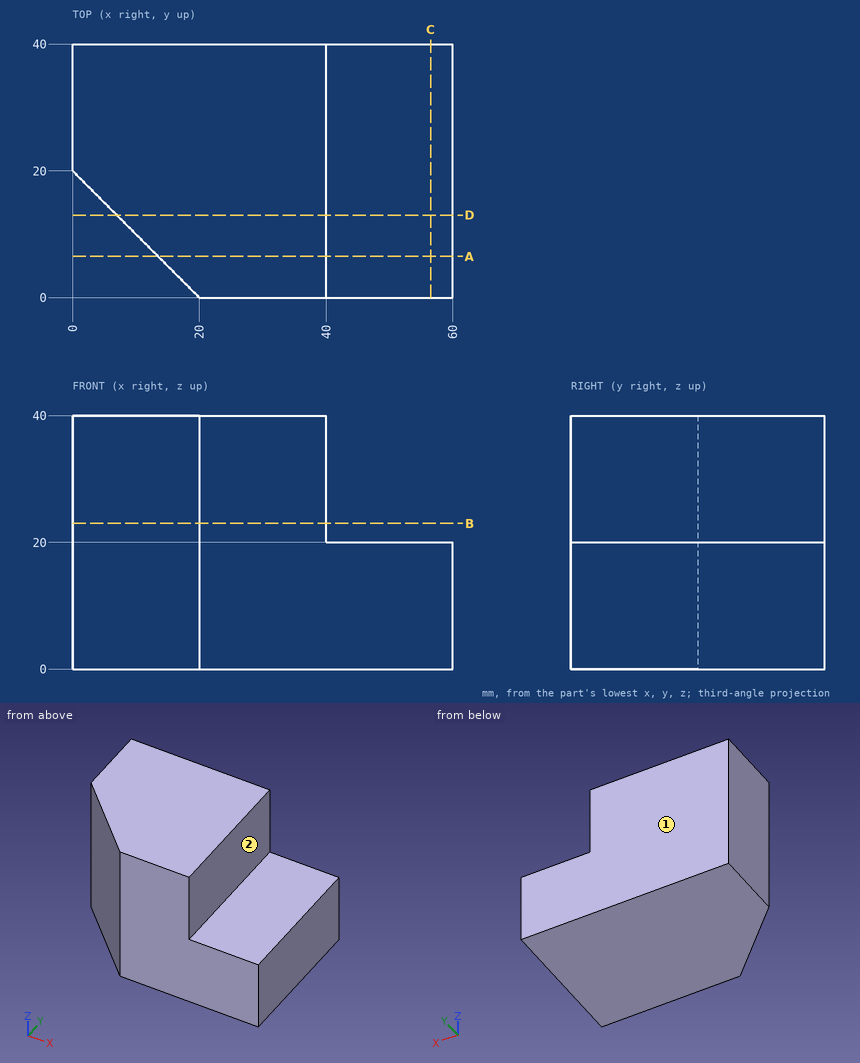
Could you check a few things on this drawing? It's one solid part, dimensions in mm from its lowest x, y, z. A direction names the side the tool comes from. Round coordinates to 2 decimals unless told otherwise and drop trailing zeros. Write each loop counter-clockwise with the first axis right and the second up, starting at its lowest first coordinate (ties: lowest second). Pieces come first, ordered by that corner, then holes. Notation, with made-up numbers: (-11.5, -3.5) -> (12.5, -3.5) arc R34 cw to (12.5, 27.5) -> close; hole circle Ø3 at (4.25, 21.5). An arc over 180 degrees is marked (long way). One line per question, with ' | ' between items. Start each with the question number.
1) I need wall thicknesses on line 1 (Z direction, x = 44, y = 15); line 2 (X direction, y = 33, z = 32); line 3 (Y direction, x = 4.5, z = 4). Which ranges of each line are inside material? Lowest first, please. Write a range as [from, to].
2) Suppose I cut it at A-A on y = 6.5. Write out the boundary of the cut face in (x, z).
3) Suppose I cut it at B-B on z = 23. Write out the boundary of the cut face in (x, y).
4) Suppose I cut it at C-C on x = 56.5. Write out the boundary of the cut face in (y, z), then the cut area to 3 significant figures.
5) I'm going to push flat-ended pins straight in: P1, Ø3, axis at x = 15.5, z = 22.5, coming from the -Y side; P2, Ø6, axis at x = 47, y = 15, coming from the +Z side; P3, Ø2, axis at x = 42.5, z = 35.5, coming from the -Y side; P4, Ø1, axis at x = 37, z = 10, coming from the -Y side. Where does each tip first touch, or does it pass through?
6) Suppose I cut it at D-D on y = 13. Write out the boundary of the cut face in (x, z).
7) On a 3-axis mill with a long thin cutter (end or side, diameter ignored), from which of +Z, -Z, +X, -X, +Y, -Y can I reach the whole of each face in a straight line? I mean the marked faces 1 and 2. Say none if no direction works.
Return value:
1) line 1: z = [0, 20] | line 2: x = [0, 40] | line 3: y = [15.5, 40]
2) outline: (13.5, 0) -> (60, 0) -> (60, 20) -> (40, 20) -> (40, 40) -> (13.5, 40) -> close
3) outline: (0, 20) -> (20, 0) -> (40, 0) -> (40, 40) -> (0, 40) -> close
4) outline: (0, 0) -> (40, 0) -> (40, 20) -> (0, 20) -> close | area: 800 mm2
5) P1: stops at y = 3 | P2: stops at z = 20 | P3: passes through | P4: stops at y = 0
6) outline: (7, 0) -> (60, 0) -> (60, 20) -> (40, 20) -> (40, 40) -> (7, 40) -> close
7) face 1: +Z, -Z, +X, -X, +Y | face 2: +Z, +X, +Y, -Y
